```python
from build123d import *

# Parameters (mm, degrees)
SKETCH1_R           = 2.25
SKETCH1_R_2         = 1.6
BOSS_EXTRUDE1_DEPTH = 25
SKETCH2_R           = 2.25
BOSS_EXTRUDE2_DEPTH = 1.5
SKETCH3_W           = 10
SKETCH3_H           = 2
BOSS_EXTRUDE3_DEPTH = 1.5
SKETCH4_W           = 2
SKETCH4_H           = 2
BOSS_EXTRUDE4_DEPTH = 0.8
SKETCH5_W           = 2.8
SKETCH5_H           = 2
BOSS_EXTRUDE5_DEPTH = 0.7


with BuildPart() as part:
    # Sketch1 → Boss-Extrude1 (new body)
    with BuildSketch(Plane.XY):
        Circle(SKETCH1_R)
        Circle(SKETCH1_R_2, mode=Mode.SUBTRACT)
    extrude(amount=-BOSS_EXTRUDE1_DEPTH)

    # Sketch2 → Boss-Extrude2 (add)
    with BuildSketch(Plane(origin=(0, 0, -25), x_dir=(-1, 0, 0), z_dir=(0, 0, -1))):
        with Locations(Location((0, 0, 0), (0, 0, 180))):
            Circle(SKETCH2_R)
    extrude(amount=BOSS_EXTRUDE2_DEPTH)

    # Sketch3 → Boss-Extrude3 (add)
    with BuildSketch(Plane(origin=(0, 0, -26.5), x_dir=(-1, 0, 0), z_dir=(0, 0, -1))):
        Rectangle(SKETCH3_W, SKETCH3_H)
    extrude(amount=BOSS_EXTRUDE3_DEPTH)

    # Sketch4 → Boss-Extrude4 (add)
    with BuildSketch(Plane(origin=(0, 0, -28), x_dir=(-1, 0, 0), z_dir=(0, 0, -1))):
        with Locations((-4, 0)):
            Rectangle(SKETCH4_W, SKETCH4_H)
        with Locations((4, 0)):
            Rectangle(SKETCH4_W, SKETCH4_H)
    extrude(amount=BOSS_EXTRUDE4_DEPTH)

    # Sketch5 → Boss-Extrude5 (add)
    with BuildSketch(Plane(origin=(0, 0, -28.8), x_dir=(-1, 0, 0), z_dir=(0, 0, -1))):
        with Locations((-3.6, 0)):
            Rectangle(SKETCH5_W, SKETCH5_H)
        with Locations((3.6, 0)):
            Rectangle(SKETCH5_W, SKETCH5_H)
    extrude(amount=BOSS_EXTRUDE5_DEPTH)


solid = part.part
```
CAD build for the part. Positions are in the model's coordinates, mm. A direction names the side the tool comes from. Round coordinates to 2 decimals unless told otherwise and drop trailing zeros. Order: outer loops, then holes, each group sorted by start corner. A loop starts at its lowest first (then second) coordinate and runs counter-clockwise, first axis right, second up.
Q1. Wall check: L1, parallel to Z at x = 2.75, y = 0.6; L2, parallel to Y at x = 0, z = -10.75; L3, parallel to Z at x = -3.25, y = -0.8. Give the ranges that are in metal, low to high.
Q2. Which spindle directions (+Z, -Z, +X, -X, +Y, -Y) get a long thin tool onto all of the face, cutting with end or side? Do faces 1 (the flat face through (-4, 0, -29.5)), 2 (the flat face through (0.1, -1, -27.6)), 3 (the flat face through (0, 0, -25)), 4 (the flat face through (0, 1.5, -26.5)), 5 (the flat face through (3, 0, -28.4)). Say none if no direction does.
Q3. Two-plate mould, pull along Z, no slides. Class faces 6 (the flat face through (4, 0, -29.5)), 7 (the flat face through (-2, 0, 0)), 8 (the flat face through (5, 0, -28)), 9 (the flat face through (0, 0, -28)): pulls with the +Z half, pulls with the -Z half, needs draft (parallel to the pull), parting line crosses it, or undercut.
Q4. Slice it at A-A (z = -20.75). Write the cut outline in (x, y), and give its area (3 significant figures).
Q5. Slice it at C-C (x = 0). Write the cut outline in (y, z).
Q6. Slice it at B-B (y = 0). Write the cut outline in (x, z), and give its area (3 significant figures).
Q7. Slice it at D-D (z = -25.5). Write the cut outline in (x, y), and give its area (3 significant figures).
Q8. Drop flat-ended pins along their axis: pin 1 (1 mm diameter, centred on x = 0, y = 0, fed in from +Z); pin 2 (1 mm diameter, centred on x = -4, y = 0.5, fed in from +Z); pin 3 (1.6 mm diameter, centred on x = 0, y = -0.5, fed in from -Z). Give the stop position or say it passes through.
Results below:
1. L1: z = -29.5 to -28.8, -28 to -26.5
1. L2: y = -2.25 to -1.6, 1.6 to 2.25
1. L3: z = -29.5 to -26.5
2. face 1: -Z, +X, -X, +Y, -Y
2. face 2: -Z, +X, -X, -Y
2. face 3: +Z
2. face 4: -Z, +X, -X, +Y
2. face 5: +Y, -Y
3. face 6: pulls with the -Z half
3. face 7: pulls with the +Z half
3. face 8: needs draft
3. face 9: undercut
4. outline: circle Ø4.5 at (0, 0); hole circle Ø3.2 at (0, 0)
4. area: 7.86 mm2
5. outline: (-2.25, -26.5) - (-1, -26.5) - (-1, -28) - (1, -28) - (1, -26.5) - (2.25, -26.5) - (2.25, 0) - (1.6, 0) - (1.6, -25) - (-1.6, -25) - (-1.6, 0) - (-2.25, 0) - close
6. outline: (-5, -29.5) - (-2.2, -29.5) - (-2.2, -28.8) - (-3, -28.8) - (-3, -28) - (3, -28) - (3, -28.8) - (2.2, -28.8) - (2.2, -29.5) - (5, -29.5) - (5, -26.5) - (2.25, -26.5) - (2.25, 0) - (1.6, 0) - (1.6, -25) - (-1.6, -25) - (-1.6, 0) - (-2.25, 0) - (-2.25, -26.5) - (-5, -26.5) - close
6. area: 61.4 mm2
7. outline: circle Ø4.5 at (0, 0)
7. area: 15.9 mm2
8. pin 1: stops at z = -25
8. pin 2: stops at z = -26.5
8. pin 3: stops at z = -28
